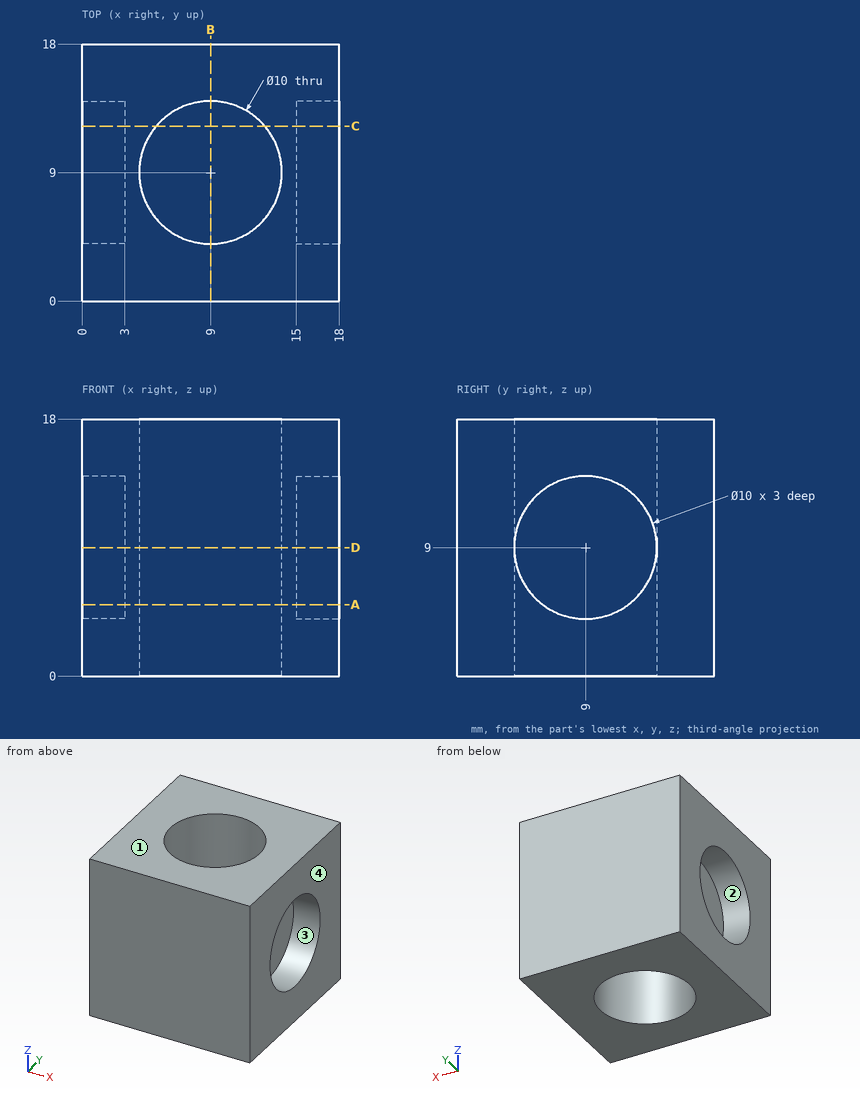
Input: dimensioned drawing with shaded views. Units: mm. Origin: part minimum x, y, z. Coordinates: 2 decimals unless noted, no trailing zeros. Loops run counter-clockwise (first coordinate to the right, second up) from the corner with the lowest first, then second, coordinate; pieces in that order, holes last.
Q1. Section D-D, the plane z = 9. Return the cut outline in (x, y).
Results are:
outline: (0, 0) - (18, 0) - (18, 4) - (15, 4) - (15, 14) - (18, 14) - (18, 18) - (0, 18) - (0, 14) - (3, 14) - (3, 4) - (0, 4) - close; hole circle Ø10 at (9, 9)
Q2. Line query: line 1 along Z through (x, y) = (17.3, 9); line 2 along X through (y, z) = (9.25, 14.5); line 3 along Y through (x, z) = (6.25, 11.25). Output: solid intervals per line, ascending.
Results are:
line 1: z = 0 to 4, 14 to 18
line 2: x = 0 to 4.01, 13.99 to 18
line 3: y = 0 to 4.82, 13.18 to 18
Q3. Contact query for flat-ended pins moving along their axis: pin 1 (8 mm diameter, centred on y = 9, z = 8.5, fed in from +X); pin 2 (6 mm diameter, centred on y = 9, z = 9, fed in from -X); pin 3 (9 mm diameter, centred on x = 9, y = 9, fed in from +Z). Output: stop coordinate, or through.
Results are:
pin 1: stops at x = 15
pin 2: stops at x = 3
pin 3: passes through
Q4. Section A-A, the plane z = 5. Return the cut outline in (x, y).
Results are:
outline: (0, 0) - (18, 0) - (18, 6) - (15, 6) - (15, 12) - (18, 12) - (18, 18) - (0, 18) - (0, 12) - (3, 12) - (3, 6) - (0, 6) - close; hole circle Ø10 at (9, 9)
Q5. Section B-B, the plane x = 9. Return the cut outline in (y, z), and give its area (3 significant figures).
Results are:
outline: (0, 0) - (4, 0) - (4, 18) - (0, 18) - close; (14, 0) - (18, 0) - (18, 18) - (14, 18) - close
area: 144 mm2
Q6. Mould query, pull axis Z, two halves, no side actions, for the marked faces 1, 2, 3 and 4. Classes: +Z half, -Z half, draft (parallel to the pull), parting line (faces both ways), or undercut.
Results are:
face 1: +Z half
face 2: undercut
face 3: undercut
face 4: draft
Q7. Section C-C, the plane y = 12.25. Return the cut outline in (x, z).
Results are:
outline: (0, 0) - (5.2, 0) - (5.2, 18) - (0, 18) - (0, 12.8) - (3, 12.8) - (3, 5.2) - (0, 5.2) - close; (12.8, 0) - (18, 0) - (18, 5.2) - (15, 5.2) - (15, 12.8) - (18, 12.8) - (18, 18) - (12.8, 18) - close
